Autodesk Fusion 360 part; units mm, degrees
sketch "Sketch4" plane through (0, 0, 0) normal (0, 0, 1) x (1, 0, 0)
  circle A0 centre (-30.1021, 33.9333) radius 30
  circle A1 centre (30.8979, 33.9333) radius 30
  circle A2 centre (0.3979, -19.0667) radius 30
  circle A3 centre (-60.6021, -19.0667) radius 30
  line L0 (-84.1021, 5.9333) -> (-84.1021, 6.9333)
  line L1 (27.3979, -43.0667) -> (26.9, -43.0667)
  circle A4 centre (0.3979, 86.9333) radius 30
  circle A5 centre (-60.6021, 86.9333) radius 30
  line L2 (-88.6021, 114.9333) -> (58.8979, 114.9333)
  line L3 (58.8979, 114.9333) -> (58.8979, -47.0667)
  line L4 (58.8979, -47.0667) -> (-88.6021, -47.0667)
  line L5 (-88.6021, -47.0667) -> (-88.6021, 114.9333)
  line L6 (-88.6021, 58.9333) -> (-58.1021, 58.9333)
  line L7 (-58.1021, 58.9333) -> (-58.1021, 8.9333)
  line L8 (-58.1021, 8.9333) -> (-88.6021, 8.9333)
  line L9 (-88.6021, 8.9333) -> (-88.6021, 58.9333)
  line L10 (58.8979, 61.9333) -> (28.3979, 61.9333)
  line L11 (28.3979, 61.9333) -> (28.3979, 114.9333)
  line L12 (28.3979, 114.9333) -> (58.8979, 114.9333)
  line L13 (58.8979, 114.9333) -> (58.8979, 61.9333)
  line L14 (58.8979, 5.9333) -> (28.3979, 5.9333)
  line L15 (28.3979, 5.9333) -> (28.3979, -47.0667)
  line L16 (28.3979, -47.0667) -> (58.8979, -47.0667)
  line L17 (58.8979, -47.0667) -> (58.8979, 5.9333)
  dimension "d15" = 60
  dimension "d16" = 60
  dimension "d17" = 60
  dimension "d18" = 60
  dimension "d19" = 61
  dimension "d23" = 61
  dimension "d24" = 30.5
  dimension "d25" = 53
  dimension "d46" = 60
  dimension "d47" = 60
  dimension "d48" = 61
  dimension "d49" = 53
  dimension "d50" = 30.5
  dimension "d53" = 28
  dimension "d54" = 28
  dimension "d55" = 28
  dimension "d56" = 28
  dimension "d57" = 28
  dimension "d58" = 28
  dimension "d59" = 28
  dimension "d60" = 28
  dimension "d61" = 28
  dimension "d62" = 28
  dimension "d63" = 28
  dimension "d64" = 28
extrude "Extrude6" add sketch "Sketch4" along normal blind 4 contours A0 L7 | A0 A1 A2 A3 A4 A5 L2 L4 L7 L11 L15 | A5 L2 L5 L6 L7 | A3 L4 L5 L7 L8 | A5 L5 L6 | A3 L5 L8 | A5 L2 L5 | A4 L2 L11 | A3 L4 L5 | A2 L4 L15 | A4 L2 L11 | A2 L4 L15 | A1 L3 L10 L11 L14 L15 | A1 L3 L10 | A1 L3 L14 picked at (-22.751, 30.3432)
extrude "Extrude7" add sketch "Sketch4" along normal blind 116 contours A0 A1 A2 A3 A4 A5 L2 L4 L7 L11 L15 | A5 L5 L6 | A3 L5 L8 | A5 L2 L5 | A3 L4 L5 | A4 L2 L11 | A2 L4 L15 | A1 L3 L10 | A1 L3 L14 picked at (22.8223, 111.3226) picked at (22.8223, -43.4561)
fillet "Fillet1" radius 5 8 edges at (28.3979, -47.0667, 58) (58.8979, 5.9333, 58) (58.8979, 61.9333, 58) (28.3979, 114.9333, 58) (-88.6021, 114.9333, 58) (-88.6021, 58.9333, 58) (-88.6021, 8.9333, 58) (-88.6021, -47.0667, 58)
Check sheet for the modelled part. Datum: model origin and axes. Units: mm. A direction names the side the tool comes from. Coordinates: 2 decimals unless noted, no trailing zeros. Write each loop counter-clockwise with the first axis right and the second up, starting at its lowest first coordinate (ties: lowest second). Pieces come first, ordered by that corner, then holes.
Item 1: Depth check by flat-ended pin: pin 1 Ø17.5 at (x, y) = (-12.5, -20) entering from +Z; pin 2 Ø3 at (y, z) = (27.5, 53.5) entering from -X; pin 3 Ø12 at (y, z) = (50, 75) entering from -X; pin 4 Ø12 at (x, z) = (-6, 37) entering from +Y. Enter the tip coordinate at first touch or a pass-through.
Numbers:
pin 1: stops at z = 4
pin 2: stops at x = -1.17
pin 3: stops at x = -58.1
pin 4: stops at y = 114.93
Item 2: Mould release check, pull along X, two halves, no side actions. Record for faces 3 (the face through (-81.94, 2.02, 59.22)), 4 (the face through (-84, -42, 116)), 5 (the face through (57.4, 60.5, 57.2)), 6 (the face through (21.73, -40.16, 59.22)): released by +X, released by -X, zero draft, split by the parting line, or undercut.
Numbers:
face 3: undercut
face 4: zero draft
face 5: released by +X
face 6: undercut
Item 3: Scan lines: probe 1 along Y at (x, z) = (-19.5, 74); probe 2 along Y at (x, z) = (-25.5, 22); probe 3 along X at (y, z) = (68.5, 72.5). Record each from-to range of solid material in increasing order.
Numbers:
probe 1: y = -47.07 to -41.52, 3.38 to 5.87, 62 to 64.48, 109.38 to 114.93
probe 2: y = -47.07 to -34.21, -3.92 to 4.29, 63.58 to 71.79, 102.08 to 114.93
probe 3: x = -88.6 to -84.27, -36.93 to -23.27, 24.07 to 28.4
Item 4: Cross-section at D-D on x = 34. Record the boundary of the cut face in (y, z).
Numbers:
outline: (5.93, 0) - (61.93, 0) - (61.93, 4) - (5.93, 4) - close
Item 5: Cross-section at C-C on y = 90.5. Record the boundary of the cut face in (x, z).
Numbers:
outline: (-88.6, 0) - (28.4, 0) - (28.4, 4) - (-29.39, 4) - (-29.39, 116) - (-30.81, 116) - (-30.81, 4) - (-88.6, 4) - close
Item 6: Cross-section at A-A on x = 19. Record the boundary of the cut face in (y, z), then the cut area to 3 significant figures.
Numbers:
outline: (-47.07, 0) - (114.93, 0) - (114.93, 116) - (110.47, 116) - (110.47, 4) - (63.4, 4) - (63.4, 116) - (61.47, 116) - (61.47, 4) - (6.39, 4) - (6.39, 116) - (4.47, 116) - (4.47, 4) - (-42.6, 4) - (-42.6, 116) - (-47.07, 116) - close
area: 2,080 mm2
Item 7: Cross-section at B-B on z = 36.5. Count the separate pieces of the cut face and the enclosed holes in it, then the cut area to 3 significant figures.
Numbers:
separate pieces: 9
enclosed holes: 0
area: 2,500 mm2
Item 8: Access from +Z, -Z, +X, -X, +Y, -Y to the whole of each face (thin tool, end or side, straight path). Record for faces 1 (the face through (-88.602, -35, 57)), 2 (the face through (-81.94, 108.02, 59.22)).
Numbers:
face 1: +Z, -Z, -X, +Y, -Y
face 2: +Z
